Source: three-view drawing plus pictorial views. Frame: mm from the lowest corner of the part. Give positions to 0.01 mm unless a question says otherwise; leave off trailing zeros. Order: outer loops, then holes, each group sorted by start corner. A loop starts at its lowest first (then second) coordinate and runs counter-clockwise, first axis right, second up. Notation, with made-up numbers: (47.25, 76) - (74.25, 76) arc R19 cw to (74.25, 80) - close; hole circle Ø11 at (27, -22). An arc over 180 degrees is marked (long way). Use CSV: the item, a comma, the result in double quotes.
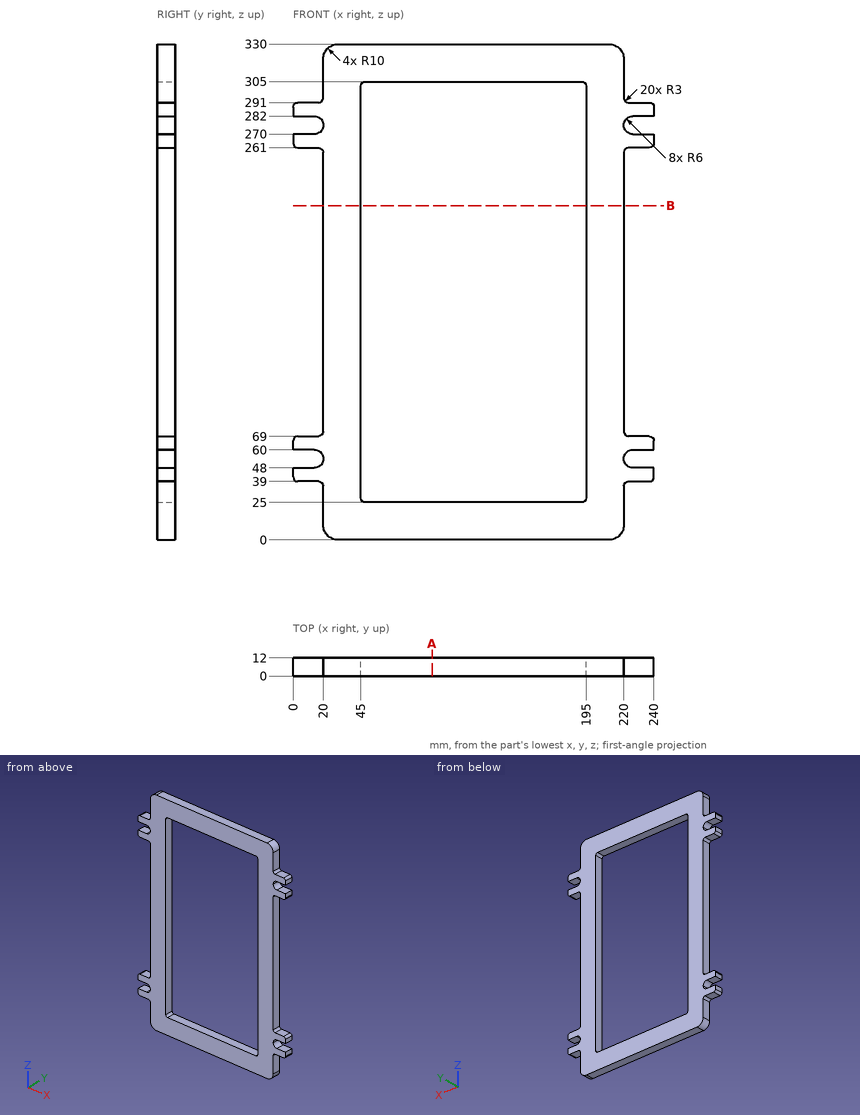
Item 1: Section A-A on x = 92.5. Return the cut outline in (y, z).
Filled in:
outline,"(0, 0) - (12, 0) - (12, 25) - (0, 25) - close; (0, 305) - (12, 305) - (12, 330) - (0, 330) - close"
Item 2: Section B-B on z = 222.5. Return the cut outline in (x, y), then the cut area to 3 significant figures.
Filled in:
outline,"(20, 0) - (45, 0) - (45, 12) - (20, 12) - close; (195, 0) - (220, 0) - (220, 12) - (195, 12) - close"
area,"600 mm2"
Item 3: Material intervals for line 1 (Z direction, x = 90, y = 3.5); line 2 (Z direction, x = 11.5, y = 1); line 3 (X direction, y = 7, z = 196.5), sorted ascending. Write a range as from..to.
Filled in:
line 1,"z = 0..25, 305..330"
line 2,"z = 39..48, 60..69, 261..270, 282..291"
line 3,"x = 20..45, 195..220"
Item 4: First-contact query: pin 1 (6 mm diameter, centred on x = 6.5, y = 9, fed in from -Z); pin 2 (6 mm diameter, centred on y = 9, z = 56, fed in from -X); pin 3 (1 mm diameter, centred on y = 7.5, z = 189, fed in from +X). Flat tips, straight axial feed; report the tip coordinate or a pass-through.
Filled in:
pin 1,"stops at z = 39"
pin 2,"stops at x = 17.32"
pin 3,"stops at x = 220"
